from build123d import *

# Parameters (mm, degrees)
SKETCH1_W               = 142.5
SKETCH1_H               = 172.5
BOSS_EXTRUDE1_DEPTH     = 4
CUT_EXTRUDE1_DEPTH      = 224.889481665
CUT_EXTRUDE1_DEPTH_BACK = 224.889481665
SKETCH2_R               = 2.25
CUT_EXTRUDE2_DEPTH      = 224.889481665
CUT_EXTRUDE2_DEPTH_BACK = 4.5
SKETCH3_R               = 3.75


with BuildPart() as part:
    # Sketch1 → Boss-Extrude1 (new, symmetric)
    with BuildSketch(Plane(origin=(0, 0, 0), x_dir=(1, 0, 0), z_dir=(0, 1, 0))):
        with Locations((71.25, 86.25)):
            Rectangle(SKETCH1_W, SKETCH1_H)
    extrude(amount=BOSS_EXTRUDE1_DEPTH, both=True)

    # Sketch2 → Cut-Extrude1 (cut, two sides: drawn at the far end of the back side and taken through both)
    with BuildSketch(Plane(origin=(0, 4, 0), x_dir=(1, 0, 0), z_dir=(0, 1, 0)).offset(-CUT_EXTRUDE1_DEPTH_BACK)):
        with Locations(Location((7.5, 165, 0), (0, 0, 270))):
            Circle(SKETCH2_R)
        with Locations(Location((135, 165, 0), (0, 0, 270))):
            Circle(SKETCH2_R)
        with Locations(Location((135, 7.5, 0), (0, 0, 270))):
            Circle(SKETCH2_R)
        with Locations(Location((7.5, 7.5, 0), (0, 0, 270))):
            Circle(SKETCH2_R)
    extrude(amount=CUT_EXTRUDE1_DEPTH + CUT_EXTRUDE1_DEPTH_BACK, mode=Mode.SUBTRACT)

    # Sketch3 → Cut-Extrude2 (cut, two sides: drawn at the far end of the back side and taken through both)
    with BuildSketch(Plane(origin=(0, 4, 0), x_dir=(1, 0, 0), z_dir=(0, 1, 0)).offset(-CUT_EXTRUDE2_DEPTH_BACK)):
        with Locations(Location((7.5, 165, 0), (0, 0, 90))):
            Circle(SKETCH3_R)
        with Locations(Location((135, 165, 0), (0, 0, 90))):
            Circle(SKETCH3_R)
        with Locations(Location((135, 7.5, 0), (0, 0, 90))):
            Circle(SKETCH3_R)
        with Locations(Location((7.5, 7.5, 0), (0, 0, 90))):
            Circle(SKETCH3_R)
    extrude(amount=CUT_EXTRUDE2_DEPTH + CUT_EXTRUDE2_DEPTH_BACK, mode=Mode.SUBTRACT)


solid = part.part
Input: part model. Units: mm. Frame: model coordinates. A direction names the side the tool comes from. Give positions to 0.01 mm unless a question says otherwise; leave off trailing zeros. Order: outer loops, then holes, each group sorted by start corner. A loop starts at its lowest first (then second) coordinate and runs counter-clockwise, first axis right, second up. Notation, with made-up numbers: (82.25, -1.5) - (131.25, -1.5) arc R21 cw to (131.25, 16.5) - close; hole circle Ø10 at (61, 75). An arc over 180 degrees is marked (long way). Answer as a JSON object with one key per item and string values. Group by question number.
Q1. First-contact query: pin 1 Ø3.5 at (x, z) = (7.5, -165) entering from +Y; pin 2 Ø2 at (x, z) = (6, -166.5) entering from +Y. Flat tips, straight axial feed; report the tip coordinate or a pass-through.
Q2. Mould query, pull axis X, two halves, no side actions, for faces 3 (the face through (142.5, 0, -85)), 4 (the face through (0, 0, -85)), 5 (the face through (138.66, 1.72, -164.19)), 6 (the face through (70, 0, -172.5)). Classes: pulls with the +X half, pulls with the -X half, needs draft (parallel to the pull), parting line crosses it, or undercut.
Q3. Line query: probe 1 along X at (y, z) = (2.9, -165); probe 2 along Z at (x, y) = (7.5, -1.8); probe 3 along X at (y, z) = (-3.1, -7.5). Output: solid intervals per line, ascending.
Q4. Cut plane A-A, the plane z = -165. Output: boundary loops of the cut face in (x, y).
Q5. Set-up query: faces 1 (the face through (132.804, -2.274, -7.988)), 2 (the face through (138.66, 1.72, -6.69)). Return all of +Z, -Z, +X, -X, +Y, -Y with unobstructed straight access to the full face (end or side cutting, diameter ignored); none if empty.
Q6. Cut plane B-B, the plane x = 135. Output: boundary loops of the cut face in (y, z).
Results:
{
 "1": {"pin 1": "through", "pin 2": "y = -0.5"},
 "2": {"face 3": "pulls with the +X half", "face 4": "pulls with the -X half", "face 5": "undercut", "face 6": "needs draft"},
 "3": {"probe 1": "0 to 3.75, 11.25 to 131.25, 138.75 to 142.5", "probe 2": "-172.5 to -167.25, -162.75 to -9.75, -5.25 to 0", "probe 3": "0 to 5.25, 9.75 to 132.75, 137.25 to 142.5"},
 "4": {"outline": "(0, -4) - (5.25, -4) - (5.25, -0.5) - (3.75, -0.5) - (3.75, 4) - (0, 4) - close; (9.75, -4) - (132.75, -4) - (132.75, -0.5) - (131.25, -0.5) - (131.25, 4) - (11.25, 4) - (11.25, -0.5) - (9.75, -0.5) - close; (137.25, -4) - (142.5, -4) - (142.5, 4) - (138.75, 4) - (138.75, -0.5) - (137.25, -0.5) - close"},
 "5": {"face 1": "+Y, -Y", "face 2": "+Y"},
 "6": {"outline": "(-4, -172.5) - (4, -172.5) - (4, -168.75) - (-0.5, -168.75) - (-0.5, -167.25) - (-4, -167.25) - close; (-4, -162.75) - (-0.5, -162.75) - (-0.5, -161.25) - (4, -161.25) - (4, -11.25) - (-0.5, -11.25) - (-0.5, -9.75) - (-4, -9.75) - close; (-4, -5.25) - (-0.5, -5.25) - (-0.5, -3.75) - (4, -3.75) - (4, 0) - (-4, 0) - close"}
}
